```python
from build123d import *

# Parameters (mm, degrees)
F0_W     = 85.5472
F0_H     = 47.498
F0_W_2   = 69.85
F0_H_2   = 31.623
F1_DEPTH = 10.16
F2_W     = 6.35
F2_H     = 6.35
F2_R     = 1.35255
F3_DEPTH = 5.08
F4_R     = 2.54
F5_W     = 76.581
F5_H     = 38.227
F5_W_2   = 69.85
F5_H_2   = 31.623
F6_DEPTH = 5.08
F7_R     = 2.54


with BuildPart() as f1:
    # F0 (on Top) → F1 (new body)
    with BuildSketch(Plane.XY):
        Rectangle(F0_W, F0_H)
        Rectangle(F0_W_2, F0_H_2, mode=Mode.SUBTRACT)
    extrude(amount=F1_DEPTH)

    # F2 (on face) → F3 (join)
    with BuildSketch(Plane.XY.offset(10.16)):
        with Locations((-31.75, -12.6365)):
            Rectangle(F2_W, F2_H)
        with Locations((-31.75, -12.6365)):
            Circle(F2_R, mode=Mode.SUBTRACT)
        with Locations((31.75, 12.6365)):
            Rectangle(F2_W, F2_H)
        with Locations((31.75, 12.6365)):
            Circle(F2_R, mode=Mode.SUBTRACT)
    extrude(amount=-F3_DEPTH)

    # F4
    f4_edges = [f1.edges().sort_by_distance(p)[0] for p in [
        (28.575, 9.4615, 7.62),
        (-28.575, -9.4615, 7.62),
    ]]
    fillet(f4_edges, radius=F4_R)

    # F5 (on face) → F6 (cut)
    with BuildSketch(Plane(origin=(0, 0, 0), x_dir=(1, 0, 0), z_dir=(0, 0, -1))):
        Rectangle(F5_W, F5_H)
        Rectangle(F5_W_2, F5_H_2, mode=Mode.SUBTRACT)
    extrude(amount=-F6_DEPTH, mode=Mode.SUBTRACT)

    # F7
    f7_edges = [f1.edges().sort_by_distance(p)[0] for p in [
        (42.7736, -23.749, 5.08),
        (42.7736, 23.749, 5.08),
        (-42.7736, -23.749, 5.08),
        (-42.7736, 23.749, 5.08),
        (0, -23.749, 0),
        (42.7736, 0, 0),
        (0, 23.749, 0),
        (-42.7736, 0, 0),
    ]]
    fillet(f7_edges, radius=F7_R)


solid = f1.part
```
Part model, mm, in its own coordinate system. A direction names the side the tool comes from. Round coordinates to 2 decimals unless told otherwise and drop trailing zeros. Write each loop counter-clockwise with the first axis right and the second up, starting at its lowest first coordinate (ties: lowest second). Pieces come first, ordered by that corner, then holes.
Item 1: Which spindle directions (+Z, -Z, +X, -X, +Y, -Y) get a long thin tool onto all of the face, cutting with end or side? Do faces 4 (the flat face through (0, 17, 5.08)), 5 (the flat face through (33, 9.462, 8)), 6 (the flat face through (-1, -23.749, 6)). Say none if no direction does.
Results:
face 4: -Z
face 5: +Z, -Z
face 6: +Z, -Z, +X, -X, -Y
Item 2: Cut at A-A, the plane y = -4.5. Give the cut face in (x, z) (1 decimal), plus the area to 3 significant figures.
Results:
outline: (-42.8, 2.5) arc R2.5 ccw to (-40.2, 0) - (-38.3, 0) - (-38.3, 5.1) - (-34.9, 5.1) - (-34.9, 10.2) - (-42.8, 10.2) - close; (34.9, 5.1) - (38.3, 5.1) - (38.3, 0) - (40.2, 0) arc R2.5 ccw to (42.8, 2.5) - (42.8, 10.2) - (34.9, 10.2) - close
area: 123 mm2
Item 3: Cut at D-D, the plane y = 18. Give the cut face in (x, z), plus the area to 3 significant figures.
Results:
outline: (-42.77, 2.54) arc R2.54 ccw to (-40.23, 0) - (-38.29, 0) - (-38.29, 5.08) - (38.29, 5.08) - (38.29, 0) - (40.23, 0) arc R2.54 ccw to (42.77, 2.54) - (42.77, 10.16) - (-42.77, 10.16) - close
area: 477 mm2
Item 4: Cut at C-C, the plane z = 4. Give the cut face in (x, y), plus the area to 3 significant figures.
Results:
outline: (-42.77, -21.21) arc R2.54 ccw to (-40.23, -23.75) - (40.23, -23.75) arc R2.54 ccw to (42.77, -21.21) - (42.77, 21.21) arc R2.54 ccw to (40.23, 23.75) - (-40.23, 23.75) arc R2.54 ccw to (-42.77, 21.21) - close; hole (-38.29, -19.11) - (38.29, -19.11) - (38.29, 19.11) - (-38.29, 19.11) - close
area: 1,130 mm2
Item 5: Two-plate mould, pull along Y, no slides. Class faces 1 (the cylindrical face through (-42.049, 22.985, 6.403)), 2 (the flat face through (42.774, 0, 6)), 3 (the cylindrical face through (-29.339, -10.186, 7.584)): +Y half, -Y half, draft (parallel to the pull), parting line (faces both ways), or undercut.
Results:
face 1: +Y half
face 2: draft
face 3: undercut
Item 6: Drop a flat-ended pin along its axis: pin 1 Ø1.6 at (x, y) = (31.75, 12.64) entering from +Z. Give the stop position or say it passes through.
Results:
pin 1: passes through
Item 7: Cut at B-B, the plane x = 17. Give the cut face in (y, z), plus the area to 3 significant figures.
Results:
outline: (-23.75, 2.54) arc R2.54 ccw to (-21.21, 0) - (-19.11, 0) - (-19.11, 5.08) - (-15.81, 5.08) - (-15.81, 10.16) - (-23.75, 10.16) - close; (15.81, 5.08) - (19.11, 5.08) - (19.11, 0) - (21.21, 0) arc R2.54 ccw to (23.75, 2.54) - (23.75, 10.16) - (15.81, 10.16) - close
area: 125 mm2
Item 8: Probe L1, parallel to Y at x = -31.75, z = 6.7; L2, parallel to Y at x = 31.75, z = 7.9; L3, parallel to Y at x = 4, z = 3. List the from-to ranges inside material, lowest first.
Results:
L1: y = -23.75 to -13.99, -11.28 to -9.46, 15.81 to 23.75
L2: y = -23.75 to -15.81, 9.46 to 11.28, 13.99 to 23.75
L3: y = -23.75 to -19.11, 19.11 to 23.75
